from build123d import *

# Parameters (mm, degrees)
SKETCH1_R           = 2.5
BOSS_EXTRUDE2_DEPTH = 4
BOSS_EXTRUDE3_DEPTH = 11
SKETCH3_R           = 3.1
CUT_EXTRUDE1_DEPTH  = 8.5
BOSS_EXTRUDE4_START = 10
SKETCH4_R           = 10
SKETCH4_R_2         = 3.1
BOSS_EXTRUDE4_DEPTH = 10
SKETCH5_W           = 5.8
SKETCH5_H           = 2.8
CUT_EXTRUDE2_DEPTH  = 8.8
SKETCH7_R           = 1.6
CUT_EXTRUDE3_DEPTH  = 10
SKETCH13_R          = 11
CUT_EXTRUDE6_DEPTH  = 10
SKETCH14_R          = 2.25
CUT_EXTRUDE7_DEPTH  = 10
CUT_EXTRUDE8_DEPTH  = 10
SKETCH16_W          = 18
SKETCH16_H          = 44.43287335
CUT_EXTRUDE9_DEPTH  = 3
FILLET1_R           = 2


with BuildPart() as part:
    # Sketch1 → Boss-Extrude2 (new body)
    with BuildSketch(Plane(origin=(0, 0, 0), x_dir=(1, 0, 0), z_dir=(0, 1, 0))):
        with BuildLine():
            Line((-10, 0), (-60, 0))
            ThreePointArc((-60, 0), (-67.071067812, 2.928932188), (-70, 10))
            Line((-70, 10), (-70, 60))
            ThreePointArc((-70, 60), (-67.071067812, 67.071067812), (-60, 70))
            Line((-60, 70), (-10, 70))
            ThreePointArc((-10, 70), (-2.928932188, 67.071067812), (0, 60))
            Line((0, 60), (0, 10))
            ThreePointArc((0, 10), (-2.928932188, 2.928932188), (-10, 0))
        make_face()
        with Locations(Location((-50.25, 19.75, 0), (0, 0, 270))):
            Circle(SKETCH1_R, mode=Mode.SUBTRACT)
        with Locations(Location((-29.56712665, 40.43287335, 0), (0, 0, 270))):
            Circle(SKETCH1_R, mode=Mode.SUBTRACT)
    extrude(amount=BOSS_EXTRUDE2_DEPTH)

    # Sketch2 → Boss-Extrude3 (add)
    with BuildSketch(Plane(origin=(0, 4, 0), x_dir=(1, 0, 0), z_dir=(0, 1, 0))):
        with BuildLine():
            Line((-10, 0), (-60, 0))
            ThreePointArc((-60, 0), (-67.071067812, 2.928932188), (-70, 10))
            Line((-70, 10), (-70, 60))
            ThreePointArc((-70, 60), (-67.071067812, 67.071067812), (-60, 70))
            Line((-60, 70), (-10, 70))
            ThreePointArc((-10, 70), (-2.928932188, 67.071067812), (0, 60))
            Line((0, 60), (0, 10))
            ThreePointArc((0, 10), (-2.928932188, 2.928932188), (-10, 0))
        make_face()
        with BuildLine():
            Line((-3, 13), (-3, 57))
            ThreePointArc((-3, 57), (-5.928932188, 64.071067812), (-13, 67))
            Line((-13, 67), (-57, 67))
            ThreePointArc((-57, 67), (-64.071067812, 64.071067812), (-67, 57))
            Line((-67, 57), (-67, 13))
            ThreePointArc((-67, 13), (-64.071067812, 5.928932188), (-57, 3))
            Line((-57, 3), (-13, 3))
            ThreePointArc((-13, 3), (-5.928932188, 5.928932188), (-3, 13))
        make_face(mode=Mode.SUBTRACT)
    extrude(amount=BOSS_EXTRUDE3_DEPTH)

    # Sketch3 → Cut-Extrude1 (cut)
    with BuildSketch(Plane.XZ):
        with Locations(Location((-50.25, -19.75, 0), (0, 0, 270))):
            Circle(SKETCH3_R)
    extrude(amount=-CUT_EXTRUDE1_DEPTH, mode=Mode.SUBTRACT)

    # Sketch4 → Boss-Extrude4 (add)
    with BuildSketch(Plane.XZ.offset(BOSS_EXTRUDE4_START)):
        with Locations(Location((-50.25, -19.75, 0), (0, 0, 90))):
            Circle(SKETCH4_R)
        with Locations(Location((-50.25, -19.75, 0), (0, 0, 270))):
            Circle(SKETCH4_R_2, mode=Mode.SUBTRACT)
    extrude(amount=-BOSS_EXTRUDE4_DEPTH)

    # Sketch5 → Cut-Extrude2 (cut)
    with BuildSketch(Plane.XZ.offset(10)):
        with Locations((-50.25, -13.25)):
            Rectangle(SKETCH5_W, SKETCH5_H)
    extrude(amount=-CUT_EXTRUDE2_DEPTH, mode=Mode.SUBTRACT)

    # Sketch7 → Cut-Extrude3 (cut)
    with BuildSketch(Plane(origin=(-50.25, -10, -9.75), x_dir=(1, 0, 0), z_dir=(0, 0, 1))):
        with Locations((0, 5)):
            Circle(SKETCH7_R)
    extrude(amount=-CUT_EXTRUDE3_DEPTH, mode=Mode.SUBTRACT)

    # Sketch13 → Cut-Extrude6 (cut)
    with BuildSketch(Plane.XZ):
        with Locations(Location((-29.56712665, -40.43287335, 0), (0, 0, 270))):
            Circle(SKETCH13_R)
    extrude(amount=-CUT_EXTRUDE6_DEPTH, mode=Mode.SUBTRACT)

    # Sketch14 → Cut-Extrude7 (cut)
    with BuildSketch(Plane(origin=(0, 4, 0), x_dir=(1, 0, 0), z_dir=(0, 1, 0))):
        with Locations(Location((-8, 62, 0), (0, 0, 270))):
            Circle(SKETCH14_R)
        with Locations(Location((-62, 62, 0), (0, 0, 270))):
            Circle(SKETCH14_R)
        with Locations(Location((-62, 8, 0), (0, 0, 270))):
            Circle(SKETCH14_R)
        with Locations(Location((-8, 8, 0), (0, 0, 270))):
            Circle(SKETCH14_R)
    extrude(amount=-CUT_EXTRUDE7_DEPTH, mode=Mode.SUBTRACT)

    # Sketch15 → Cut-Extrude8 (cut)
    with BuildSketch(Plane.XZ):
        with BuildLine():
            ThreePointArc((-19.320175884, -36.43287335), (-18.757028167, -38.397739254), (-18.56712665, -40.43287335))
            Line((-18.56712665, -40.43287335), (-11.56712665, -40.43287335))
            ThreePointArc((-11.56712665, -40.43287335), (-11.679998346, -38.420252912), (-12.017197876, -36.43287335))
            Line((-12.017197876, -36.43287335), (-19.320175884, -36.43287335))
        make_face()
        with BuildLine():
            Line((-11.56712665, -40.43287335), (-18.56712665, -40.43287335))
            ThreePointArc((-18.56712665, -40.43287335), (-18.757028167, -42.468007445), (-19.320175884, -44.43287335))
            Line((-19.320175884, -44.43287335), (-12.017197876, -44.43287335))
            ThreePointArc((-12.017197876, -44.43287335), (-11.679998346, -42.445493788), (-11.56712665, -40.43287335))
        make_face()
    extrude(amount=-CUT_EXTRUDE8_DEPTH, mode=Mode.SUBTRACT)

    # Sketch16 → Cut-Extrude9 (cut)
    with BuildSketch(Plane.XZ):
        with Locations((-9, -22.216436675)):
            Rectangle(SKETCH16_W, SKETCH16_H)
    extrude(amount=-CUT_EXTRUDE9_DEPTH, mode=Mode.SUBTRACT)

    # Fillet1
    fillet1_edges = [part.edges().sort_by_distance(p)[0] for p in [
        (-6.008598938, 3, -44.43287335),
        (-18, 3, -18.216436675),
    ]]
    fillet(fillet1_edges, radius=FILLET1_R)


solid = part.part
The listing builds one solid part. Answer for the finished solid, in the listing's coordinates (mm). A direction names the side the tool comes from. Give positions to 0.01 mm unless a question says otherwise; leave off trailing zeros. Write each loop counter-clockwise with the first axis right and the second up, starting at its lowest first coordinate (ties: lowest second). Pieces come first, ordered by that corner, then holes. Notation, with made-up numbers: (48.25, -15.5) - (58.25, -15.5) arc R13 cw to (58.25, -6.5) - close; hole circle Ø6 at (-17, 40). An arc over 180 degrees is marked (long way). Use a Markdown table: item, result.
1. Find the intervals of material crossed by probe 1 along X at (y, z) = (1.05, -62); probe 2 along X at (y, z) = (-0.5, -19.75); probe 3 along X at (y, z) = (9.5, -25.5), in increasing order. Write a range as from..to.
Values follow:
| item | result |
|---|---|
| probe 1 | x = -69.8..-64.25, -59.75..-10.25, -5.75..-0.2 |
| probe 2 | x = -60.25..-53.35, -47.15..-40.25 |
| probe 3 | x = -70..-67, -3..0 |
2. Section C-C on x = -62 is taken. Write down the section's boundary in (y, z).
Values follow:
| item | result |
|---|---|
| outline | (0, -69.8) - (15, -69.8) - (15, -65.66) - (4, -65.66) - (4, -64.25) - (0, -64.25) - close; (0, -59.75) - (4, -59.75) - (4, -10.25) - (0, -10.25) - close; (0, -5.75) - (4, -5.75) - (4, -4.34) - (15, -4.34) - (15, -0.2) - (0, -0.2) - close |
3. Each of these flat-tipped pins is pushed along its axis until it touches: P1, Ø1, axis at x = -22.5, z = -20.5, coming from the +Y side; P2, Ø1, axis at y = -6.5, z = -25.5, coming from the +X side; P3, Ø5, axis at x = -59.5, y = -3.5, coming from the -Z side. Where does it stop, or does it pass through?
Values follow:
| item | result |
|---|---|
| P1 | stops at y = 4 |
| P2 | stops at x = -41.74 |
| P3 | stops at z = -27.13 |
4. Section A-A on z = -61 is taken. Write down the section's boundary in (x, y).
Values follow:
| item | result |
|---|---|
| outline | (-69.95, 0) - (-64.02, 0) - (-64.02, 4) - (-66.17, 4) - (-66.17, 15) - (-69.95, 15) - close; (-59.98, 0) - (-10.02, 0) - (-10.02, 4) - (-59.98, 4) - close; (-5.98, 0) - (-0.05, 0) - (-0.05, 15) - (-3.83, 15) - (-3.83, 4) - (-5.98, 4) - close |
5. A tool of negligible diameter and unlimited length cuts with its end or side. For faces 4 (the flat face through (-35, 15, -1)), 5 (the cylindrical face through (-63.99, 9.42, -64.15)), 6 (the cylindrical face through (-17.4, 2.43, -17.96)), 7 (the flat face through (-14, 2, -44.433)), 8 (the cylindrical face through (-64.196, 2.028, -8.488)), from which of +Z, -Z, +X, -X, +Y, -Y can it reach the whole face along a straight path? Write none if from no direction.
Values follow:
| item | result |
|---|---|
| face 4 | +Z, -Z, +X, -X, +Y |
| face 5 | +Y |
| face 6 | +Z, +X, -Y |
| face 7 | -Y |
| face 8 | +Y, -Y |
6. Section D-D on z = -21 is taken. Write down the section's boundary in (x, y).
Values follow:
| item | result |
|---|---|
| outline | (-70, 0) - (-60.17, 0) - (-60.17, -10) - (-53.09, -10) - (-53.09, 4) - (-67, 4) - (-67, 15) - (-70, 15) - close; (-47.41, -10) - (-40.33, -10) - (-40.33, 0) - (-18, 0) - (-18, 1) arc R2 cw to (-16, 3) - (0, 3) - (0, 15) - (-3, 15) - (-3, 4) - (-47.41, 4) - close |
7. For a pull along Z with two mould halves and no side action, classify faces 1 (the cylindrical face through (-41.378, -5.07, -15.136)), 2 (the flat face through (-42, 4, -35)), 3 (the cylindrical face through (-51.85, -4.93, -10.79)) as released by +Z, released by -Z, zero draft, split by the parting line, or undercut.
Values follow:
| item | result |
|---|---|
| face 1 | split by the parting line |
| face 2 | undercut |
| face 3 | zero draft |
8. Section B-B on y = 11.5 is taken. Write down the section's boundary in (x, z).
Values follow:
| item | result |
|---|---|
| outline | (-70, -60) arc R10 ccw to (-60, -70) - (-10, -70) arc R10 ccw to (0, -60) - (0, -10) arc R10 ccw to (-10, 0) - (-60, 0) arc R10 ccw to (-70, -10) - close; hole (-67, -57) arc R10 ccw to (-57, -67) - (-13, -67) arc R10 ccw to (-3, -57) - (-3, -13) arc R10 ccw to (-13, -3) - (-57, -3) arc R10 ccw to (-67, -13) - close |
